```python
from build123d import *

# Parameters (mm, degrees)
F1_DEPTH = 12
F2_W     = 6
F2_H     = 12.5
F3_DEPTH = 70.001
F4_R     = 1


with BuildPart() as f1:
    # F0 (on Front) → F1 (new body)
    with BuildSketch(Plane.XZ):
        Polygon((6, 30), (0, 30), (0, -30), (6, -30), (70, -15), (70, 15), align=None)
    extrude(amount=F1_DEPTH)

    # F2 (on face) → F3 (cut, through all)
    with BuildSketch(Plane.YZ.offset(70)):
        with Locations((-9, 0)):
            Rectangle(F2_W, F2_H)
    extrude(amount=-F3_DEPTH, mode=Mode.SUBTRACT)

    # F4
    f4_edges = [f1.edges().sort_by_distance(p)[0] for p in [
        (70, -6, 15),
        (6, -6, 30),
        (0, -6, 30),
        (70, -6, -15),
        (6, -6, -30),
        (0, -6, -30),
    ]]
    fillet(f4_edges, radius=F4_R)


solid = f1.part
```
Verification items for the finished model (mm, model axes). A direction names the side the tool comes from. Coordinates: 2 decimals unless noted, no trailing zeros. Order: outer loops, then holes, each group sorted by start corner. A loop starts at its lowest first (then second) coordinate and runs counter-clockwise, first axis right, second up. Notation, with made-up numbers: (-17.75, 42) -> (-9.75, 42) arc R35 cw to (-9.75, 78) -> close; hole circle Ø10 at (-28.75, -17). An arc over 180 degrees is marked (long way). Put each result on its own line as item: value. Start each with the question number.
1) Go/stop test with flat-tipped pins: pin 1 (6 mm diameter, centred on x = 40.5, z = 8.5, fed in from +Y); pin 2 (5 mm diameter, centred on x = 32.5, y = -8, fed in from -Z) (3 decimals); pin 3 (4 mm diameter, centred on x = 49, y = -3.5, fed in from -Z); pin 4 (3 mm diameter, centred on x = 9, y = -1.5, fed in from +Z). Record where each tip stops, or that it passes through.
2) Tool access check on faces 1 (the flat face through (3, -6, -30)), 2 (the flat face through (35, -9, 6.25)). Record the directions out of +Z, -Z, +X, -X, +Y, -Y that give a thin tool (end or side, any length) a straight path to the whole face; none if there is none.
3) Cross-section at C-C (x = 35). Enter the section's corners in (y, z), plus the area to 3 significant figures.
4) Material ranges on L1, parallel to Y at x = 67.5, z = -4; L2, parallel to Z at x = 18.5, y = -10.5; L3, parallel to Z at x = 33.5, y = -10.5, recorded low to high.
5) Release check for a two-part mould opening along Z. For faces 3 (the flat face through (35, -9, -6.25)), 4 (the flat face through (3, -6, 30)), 5 (the flat face through (37.23, -5.92, -22.68)) record: pulls with the +Z half, pulls with the -Z half, needs draft (parallel to the pull), parting line crosses it, or undercut.
6) Cross-section at D-D (z = 3.5). Enter the section's corners in (x, y).
7) Cross-section at A-A (y = -10.5). Enter the section's corners in (x, z).
8) Cross-section at B-B (y = -3.25). Enter the section's corners in (x, z), plus the area to 3 significant figures.
Geometry check:
1. pin 1: stops at y = 0
1. pin 2: stops at z = -24.375
1. pin 3: stops at z = -20.39
1. pin 4: stops at z = 29.65
2. face 1: -Z, +X, -X, +Y, -Y
2. face 2: +X, -X, -Y
3. outline: (-12, -23.2) -> (0, -23.2) -> (0, 23.2) -> (-12, 23.2) -> (-12, 6.25) -> (-6, 6.25) -> (-6, -6.25) -> (-12, -6.25) -> close
3. area: 482 mm^2
4. L1: y = -6 to 0
4. L2: z = -27.07 to -6.25, 6.25 to 27.07
4. L3: z = -23.55 to -6.25, 6.25 to 23.55
5. face 3: undercut
5. face 4: pulls with the +Z half
5. face 5: pulls with the -Z half
6. outline: (0, -6) -> (70, -6) -> (70, 0) -> (0, 0) -> close
7. outline: (0, -29) arc R1 ccw to (1, -30) -> (5.88, -30) arc R1 ccw to (6.11, -29.97) -> (69.23, -15.18) arc R1 ccw to (70, -14.21) -> (70, -6.25) -> (0, -6.25) -> close; (0, 6.25) -> (70, 6.25) -> (70, 14.21) arc R1 ccw to (69.23, 15.18) -> (6.11, 29.97) arc R1 ccw to (5.88, 30) -> (1, 30) arc R1 ccw to (0, 29) -> close
8. outline: (0, -29) arc R1 ccw to (1, -30) -> (5.88, -30) arc R1 ccw to (6.11, -29.97) -> (69.23, -15.18) arc R1 ccw to (70, -14.21) -> (70, 14.21) arc R1 ccw to (69.23, 15.18) -> (6.11, 29.97) arc R1 ccw to (5.88, 30) -> (1, 30) arc R1 ccw to (0, 29) -> close
8. area: 3,240 mm^2
